Read the model definition and answer for the solid it produces. Units are mm, in the model's axes. A direction names the side the tool comes from. Coordinates: 2 decimals unless noted, no trailing zeros. Loops run counter-clockwise (first coordinate to the right, second up) from the corner with the lowest first, then second, coordinate; pieces in that order, holes last.
from build123d import *

# Parameters (mm, degrees)
BOSS_EXTRUDE1_DEPTH = 1
CUT_EXTRUDE1_DEPTH  = 2
SKETCH3_W           = 13
SKETCH3_H           = 12
BOSS_EXTRUDE2_DEPTH = 2
FILLET1_R           = 1
SKETCH4_R           = 3
CUT_EXTRUDE2_DEPTH  = 4


with BuildPart() as part:
    # Sketch1 → Boss-Extrude1 (new, symmetric)
    with BuildSketch(Plane(origin=(0, 0, 0), x_dir=(1, 0, 0), z_dir=(0, 1, 0))):
        with BuildLine():
            Line((-7.381578947, 14.960526316), (-7.381578947, -65.039473684))
            ThreePointArc((-7.381578947, -65.039473684), (-2.881578947, -69.539473684), (1.618421053, -65.039473684))
            Line((1.618421053, -65.039473684), (1.618421053, 14.960526316))
            ThreePointArc((1.618421053, 14.960526316), (-2.881578947, 19.460526316), (-7.381578947, 14.960526316))
        make_face()
    extrude(amount=BOSS_EXTRUDE1_DEPTH, both=True)

    # Sketch2 → Cut-Extrude1 (cut)
    with BuildSketch(Plane(origin=(0, 1, 0), x_dir=(1, 0, 0), z_dir=(0, 1, 0))):
        with BuildLine():
            Line((-5.381578947, 14.960526316), (-5.381578947, -47.039473684))
            ThreePointArc((-5.381578947, -47.039473684), (-2.881578947, -49.539473684), (-0.381578947, -47.039473684))
            Line((-0.381578947, -47.039473684), (-0.381578947, 14.960526316))
            ThreePointArc((-0.381578947, 14.960526316), (-2.881578947, 17.460526316), (-5.381578947, 14.960526316))
        make_face()
    extrude(amount=-CUT_EXTRUDE1_DEPTH, mode=Mode.SUBTRACT)

    # Sketch3 → Boss-Extrude2 (add, symmetric)
    with BuildSketch(Plane(origin=(0, 1, 0), x_dir=(1, 0, 0), z_dir=(0, 1, 0))):
        with Locations((-2.881578947, -65.039473684)):
            Rectangle(SKETCH3_W, SKETCH3_H)
    extrude(amount=BOSS_EXTRUDE2_DEPTH, both=True)

    # Fillet1
    fillet1_edges = [part.edges().sort_by_distance(p)[0] for p in [
        (3.618421053, 1, 59.039473684),
        (-9.381578947, 1, 59.039473684),
        (-9.381578947, 1, 71.039473684),
        (3.618421053, 1, 71.039473684),
    ]]
    fillet(fillet1_edges, radius=FILLET1_R)

    # Sketch4 → Cut-Extrude2 (cut)
    with BuildSketch(Plane(origin=(0, 3, 0), x_dir=(1, 0, 0), z_dir=(0, 1, 0))):
        with Locations(Location((-2.881578947, -65.039473684, 0), (0, 0, 270))):
            Circle(SKETCH4_R)
    extrude(amount=-CUT_EXTRUDE2_DEPTH, mode=Mode.SUBTRACT)


solid = part.part
Item 1: Which of the six approach directions +Z, -Z, +X, -X, +Y, -Y give full straight-line access (tool end or side, diameter ignored) to faces 5 (the face through (1.618, 0, 23)), 6 (the face through (0, 1, 19)), 7 (the face through (3.618, 1, 65)), 8 (the face through (-2.94, 0.01, 49.54))?
Numbers:
face 5: -Z, +X, +Y, -Y
face 6: -Z, +X, -X, +Y
face 7: +Z, -Z, +X, +Y, -Y
face 8: +Y, -Y
Item 2: A cutting plane is placed at B-B on x = -4.5. Determine the outline of the cut face in (y, z), then the cut area to 3 significant figures.
Numbers:
outline: (-1, -19.16) - (1, -19.16) - (1, -16.87) - (-1, -16.87) - close; (-1, 48.94) - (1, 48.94) - (1, 59.04) - (3, 59.04) - (3, 62.51) - (-1, 62.51) - close; (-1, 67.57) - (3, 67.57) - (3, 71.04) - (-1, 71.04) - close
area: 52.6 mm2
Item 3: Determine the mould class of faces 1 (the face through (-2.75, 1.028, 62.042)), 2 (the face through (-7.382, 0, 22)), 3 (the face through (0, -1, 25)), 4 (the face through (-2.83, 0.01, -17.46)) for opening direction X: released by +X, released by -X, zero draft, split by the parting line, or undercut.
Numbers:
face 1: undercut
face 2: released by -X
face 3: zero draft
face 4: undercut
Item 4: A cutting plane is placed at A-A on z = 19. Determine the outline of the cut face in (x, y), then the cut area to 3 significant figures.
Numbers:
outline: (-7.38, -1) - (-5.38, -1) - (-5.38, 1) - (-7.38, 1) - close; (-0.38, -1) - (1.62, -1) - (1.62, 1) - (-0.38, 1) - close
area: 8.00 mm2
Item 5: A cutting plane is placed at D-D on z = 48. Determine the outline of the cut face in (x, y).
Numbers:
outline: (-7.38, -1) - (-5.19, -1) - (-5.19, 1) - (-7.38, 1) - close; (-0.57, -1) - (1.62, -1) - (1.62, 1) - (-0.57, 1) - close
Item 6: Given pin 1 (2 mm diameter, centred on y = -0.5, z = 27, fed in from -X); pin 2 (1.2 mm diameter, centred on x = -5, y = 2, fed in from -Z); pin 3 (2 mm diameter, centred on y = 0, z = 23, fed in from +X), each flat-ended and moving along its own axis, determine where each tip first touches the part or whether it passes through.
Numbers:
pin 1: stops at x = -7.38
pin 2: stops at z = 59.04
pin 3: stops at x = 1.62
Item 7: Find the intervals of material crossed by line 1 along X through (y, z) = (0, 43.5); line 2 along Z through (x, y) = (-2.75, 2.8); line 3 along Z through (x, y) = (-2.25, 0.65), in increasing order.
Numbers:
line 1: x = -7.38 to -5.38, -0.38 to 1.62
line 2: z = 59.04 to 62.04, 68.04 to 71.04
line 3: z = -19.42 to -17.38, 49.46 to 62.11, 67.97 to 71.04
Item 8: A cutting plane is placed at C-C on y = 2.4. Determine the outline of the cut face in (x, z), then the cut area to 3 significant figures.
Numbers:
outline: (-9.38, 60.04) arc R1 ccw to (-8.38, 59.04) - (2.62, 59.04) arc R1 ccw to (3.62, 60.04) - (3.62, 70.04) arc R1 ccw to (2.62, 71.04) - (-8.38, 71.04) arc R1 ccw to (-9.38, 70.04) - close; hole circle Ø6 at (-2.88, 65.04)
area: 127 mm2
